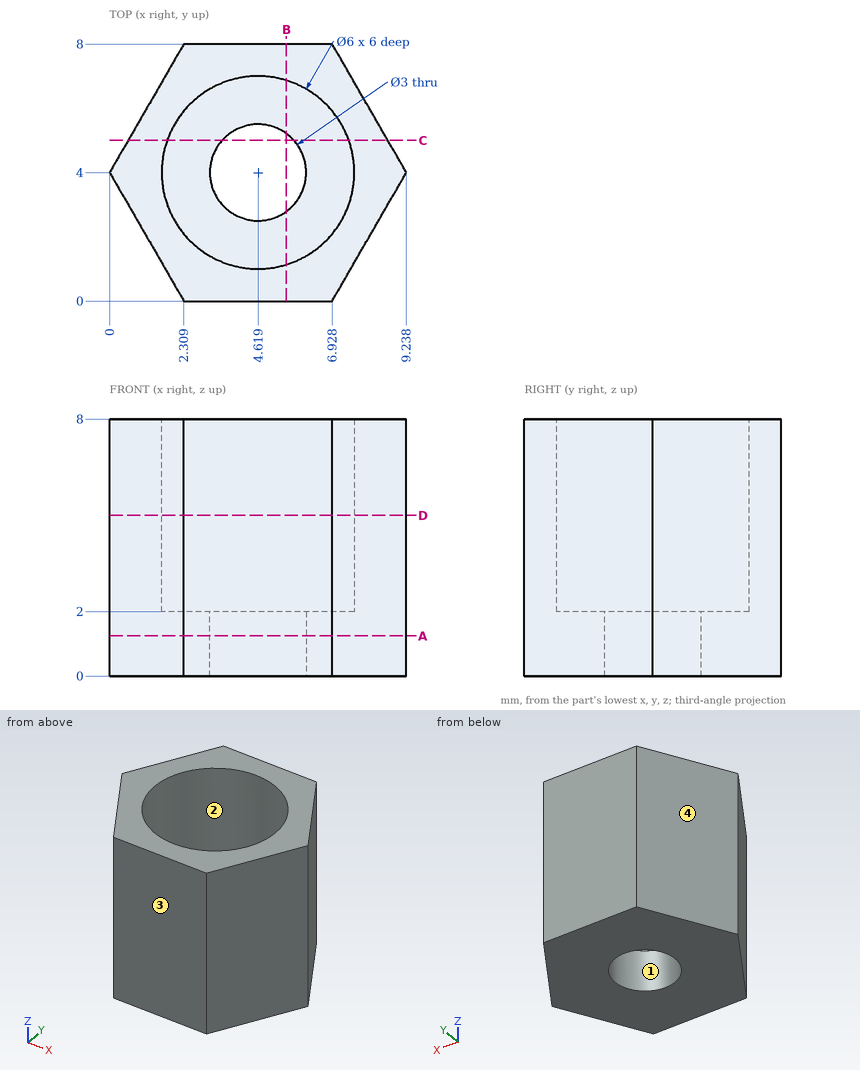
Can you work these out from the drawing? Everything is in mm from the part's minimum corner. Round coordinates to 2 decimals unless told otherwise and drop trailing zeros. Order: outer loops, then holes, each group sorted by start corner. A loop starts at its lowest first (then second) coordinate and runs counter-clockwise, first axis right, second up. Notation, with made-up numbers: (35, 46.25) - (86, 46.25) arc R29 cw to (86, 66.25) - close; hole circle Ø3 at (46, -23.75). An arc over 180 degrees is marked (long way). Answer in a Markdown table with one row per item.
(1) Suppose I cut it at B-B, the plane x = 5.5. Please give me the cut outline in (y, z).
From the geometry:
| item | result |
|---|---|
| outline | (0, 0) - (2.79, 0) - (2.79, 2) - (1.13, 2) - (1.13, 8) - (0, 8) - close; (5.21, 0) - (8, 0) - (8, 8) - (6.87, 8) - (6.87, 2) - (5.21, 2) - close |
(2) For P1, Ø4, axis at y = 1, z = 5.5, coming from the +X side; P2, Ø4, axis at y = 3, z = 6, coming from the -X side; P3, Ø1.5, axis at y = 5, z = 4.5, coming from the +X side, each with a flat end and sliding along its axis, tell me the tip position at first contact or that it passes through.
From the geometry:
| item | result |
|---|---|
| P1 | stops at x = 8.66 |
| P2 | stops at x = 0 |
| P3 | stops at x = 9.09 |
(3) If we mould it in two halves opening along X, with no side actions, what happens to the marked faces 1, 2, 3 and 4? For each: released by +X, released by -X, zero draft, split by the parting line, or undercut.
From the geometry:
| item | result |
|---|---|
| face 1 | undercut |
| face 2 | undercut |
| face 3 | zero draft |
| face 4 | released by -X |
(4) Suppose I cut it at A-A, the plane z = 1.25. Please give me the cut outline in (x, y).
From the geometry:
| item | result |
|---|---|
| outline | (0, 4) - (2.31, 0) - (6.93, 0) - (9.24, 4) - (6.93, 8) - (2.31, 8) - close; hole circle Ø3 at (4.62, 4) |
(5) Please list where these lines run through material, in increasing order: L1, parallel to X at y = 3.5, z = 7; L2, parallel to X at y = 5, z = 3.75; L3, parallel to Y at x = 4.25, z = 6. Write a range as from..to.
From the geometry:
| item | result |
|---|---|
| L1 | x = 0.29..1.66, 7.58..8.95 |
| L2 | x = 0.58..1.79, 7.45..8.66 |
| L3 | y = 0..1.02, 6.98..8 |
(6) Suppose I cut it at D-D, the plane z = 5. Please give me the cut outline in (x, y).
From the geometry:
| item | result |
|---|---|
| outline | (0, 4) - (2.31, 0) - (6.93, 0) - (9.24, 4) - (6.93, 8) - (2.31, 8) - close; hole circle Ø6 at (4.62, 4) |
(7) Suppose I cut it at C-C, the plane y = 5. Please give me the cut outline in (x, z).
From the geometry:
| item | result |
|---|---|
| outline | (0.58, 0) - (3.5, 0) - (3.5, 2) - (1.79, 2) - (1.79, 8) - (0.58, 8) - close; (5.74, 0) - (8.66, 0) - (8.66, 8) - (7.45, 8) - (7.45, 2) - (5.74, 2) - close |
